The figure shows three views and two pictorial views of one solid part (mm, origin at its lowest corner). Answer the questions. Round coordinates to 2 decimals unless told otherwise and drop trailing zeros. Write each loop counter-clockwise with the first axis right and the second up, starting at its lowest first coordinate (ties: lowest second). Pieces come first, ordered by that corner, then holes. Notation, with made-up numbers: (38, 3) -> (68, 3) arc R9 ccw to (68, 9) -> close; hole circle Ø4 at (-14, 45). An arc over 180 degrees is marked (long way). One line per item, written item: value.
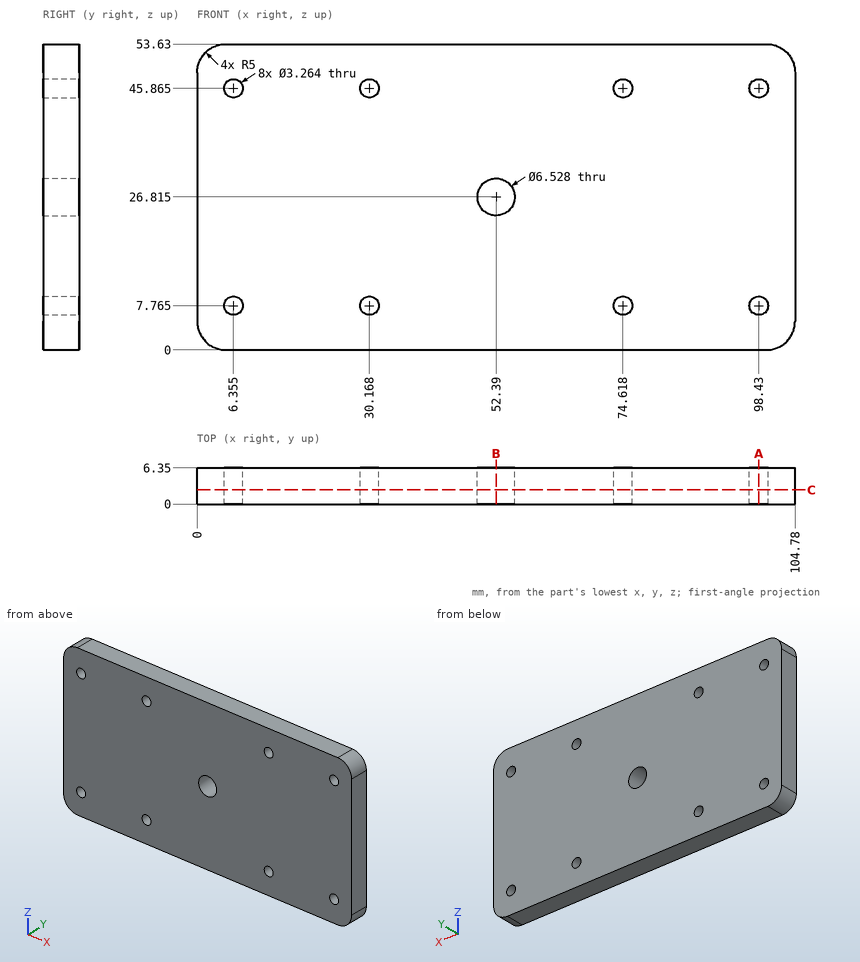
(1) Consider probe 1 along Z at (x, y) = (98.5, 5) (1 decimal); probe 2 along X at (y, z) = (1.5, 8) (1 decimal); probe 3 along Z at (x, y) = (52.39, 4). Determine where each line is inside the solid, lowest interval first.
Reported:
probe 1: z = 0 to 6.1, 9.4 to 44.2, 47.5 to 53.6
probe 2: x = 0 to 4.7, 8 to 28.6, 31.8 to 73, 76.2 to 96.8, 100 to 104.8
probe 3: z = 0 to 23.55, 30.08 to 53.63
(2) Find section C-C on y = 2.5. Give the number of separate pieces and of enclosed holes in the cut face, plus the area to 3 significant figures.
Reported:
separate pieces: 1
enclosed holes: 9
area: 5,500 mm2
(3) Find section B-B on x = 52.39. Give the vertices of the cut face in (y, z), plus the area to 3 significant figures.
Reported:
outline: (0, 0) -> (6.35, 0) -> (6.35, 23.55) -> (0, 23.55) -> close; (0, 30.08) -> (6.35, 30.08) -> (6.35, 53.63) -> (0, 53.63) -> close
area: 299 mm2
(4) Find section A-A on x = 98.43. Give the vertices of the cut face in (y, z).
Reported:
outline: (0, 0) -> (6.35, 0) -> (6.35, 6.13) -> (0, 6.13) -> close; (0, 9.4) -> (6.35, 9.4) -> (6.35, 44.23) -> (0, 44.23) -> close; (0, 47.5) -> (6.35, 47.5) -> (6.35, 53.63) -> (0, 53.63) -> close
(5) Flat-ended cylindrical pins translate along their axes: pin 1 Ø8 at (x, z) = (87, 35.5) entering from -Y; pin 2 Ø2 at (x, z) = (6.355, 7.765) entering from +Y. Find the tip coordinate at first contact, or state that the pin passes through.
Reported:
pin 1: stops at y = 0
pin 2: passes through
